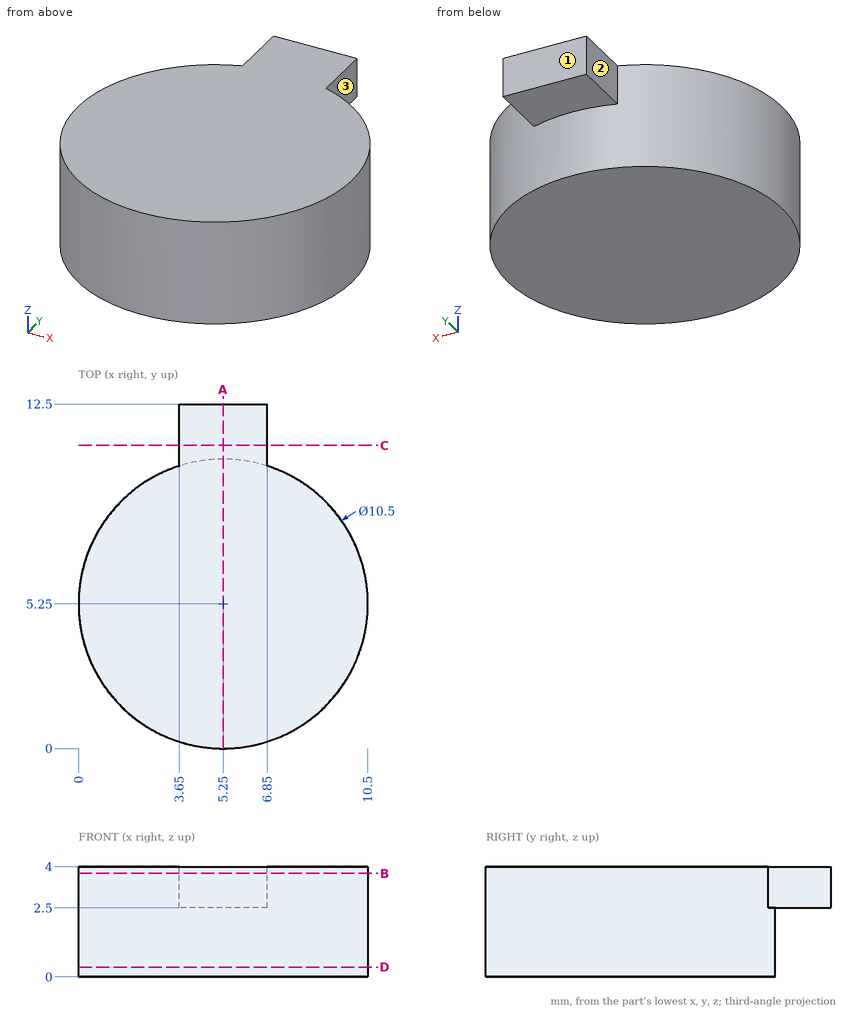
Answer from the drawing. Dimensions are ordinates in mm from the lowest x, y and z of the part. A direction names the side the tool comes from. Give positions to 0.01 mm unless a question says otherwise; leave off trailing zeros. Write each loop counter-clockwise with the first axis right and the second up, starting at its lowest first coordinate (ties: lowest second). Pieces come first, ordered by that corner, then holes. Notation, with made-up numbers: (26.5, -11) - (78.5, -11) arc R15 ccw to (78.5, 17) - close; hole circle Ø9 at (79.5, 11). An arc over 180 degrees is marked (long way). One line per item, written item: value. Start each with the question number.
1. Find section A-A (x = 5.25). Write down the section's boundary in (y, z).
2. Given pin 1 (6 mm diameter, centred on x = 9, y = 10.5, fed in from -Z); pin 2 (2 mm diameter, centred on x = 8.5, z = 3, fed in from +Y); pin 3 (0.8 mm diameter, centred on y = 11.5, z = 3.5, fed in from -X); pin 4 (1.1 mm diameter, centred on x = 6, y = 11.5, fed in from -Z), each flat-ended and moving along its own axis, determine where each tip first touches the part or whether it passes through.
3. Find section D-D (z = 0.35). Write down the section's boundary in (x, y), then the cut area to 3 significant figures.
4. For the marked faces 1, 2 and 3, determine the directions among +Z, -Z, +X, -X, +Y, -Y from which every point of the face is accessible in a straight line to the end or side of a thin tool.
5. Find section C-C (y = 11). Write down the section's boundary in (x, z), then the cut area to 3 significant figures.
6. Find section B-B (z = 3.75). Write down the section's boundary in (x, y), then the cut area to 3 significant figures.
7. Consider probe 1 along X at (y, z) = (11.25, 2.9); probe 2 along X at (y, z) = (1.5, 2.7); probe 3 along Y at (x, z) = (3, 2.75). Determine where each line is inside the solid, lowest interval first.
Geometry results:
1. outline: (0, 0) - (10.5, 0) - (10.5, 2.5) - (12.5, 2.5) - (12.5, 4) - (0, 4) - close
2. pin 1: z = 0
2. pin 2: y = 9.99
2. pin 3: x = 3.65
2. pin 4: z = 2.5
3. outline: circle Ø10.5 at (5.25, 5.25)
3. area: 86.6 mm2
4. face 1: +Z, -Z, +X, -X, +Y
4. face 2: +Z, -Z, -X, +Y
4. face 3: +Z, -Z, +X, +Y
5. outline: (3.65, 2.5) - (6.85, 2.5) - (6.85, 4) - (3.65, 4) - close
5. area: 4.80 mm2
6. outline: (3.65, 10.25) arc R5.25 ccw (long way) to (6.85, 10.25) - (6.85, 12.5) - (3.65, 12.5) - close
6. area: 93.3 mm2
7. probe 1: 3.65 to 6.85
7. probe 2: 1.58 to 8.92
7. probe 3: 0.51 to 9.99
